Autodesk Inventor part; units mm, degrees
ref_plane "YZ Plane" through (0, 0, 0) normal (1, 0, 0) x (0, 1, 0)
ref_plane "XZ Plane" through (0, 0, 0) normal (0, 1, 0) x (-1, 0, 0)
ref_plane "XY Plane" through (0, 0, 0) normal (0, 0, 1) x (1, 0, 0)
ref_plane "Work Plane1" through (0, 0, 0) normal (0, 0, 1) x (1, 0, 0)
ref_plane "Work Plane2" through (0, 0, 0) normal (0, 0, 1) x (1, 0, 0)
sketch "Sketch3" plane through (0, 0, 0) normal (0, 0, 1) x (1, 0, 0)
  circle A0 centre (-75, -25) radius 100
  circle A1 centre (-75, -25) radius 95
  point P0 (-75, -25)
  point P1 (-75, -25)
  point P2 (-75, -25)
  point P3 (-75, -25)
extrude "Extrusion3" add sketch "Sketch3" along normal blind 3 contours A0 | A1
sketch "Sketch9" plane through (0, 0, 0) normal (0, 0, -1) x (-1, 0, 0)
  line L0 (115, -125) -> (35, -125)
  line L1 (35, -105) -> (95, -105)
  line L2 (95, -105) -> (95, -85)
  line L3 (95, -85) -> (35, -85)
  line L4 (35, -85) -> (35, -105)
  line L5 (35, -105) -> (95, -85) construction
  line L6 (95, -105) -> (35, -85) construction
  arc A0 (120.4545, -114.0724) -> (120.4545, 64.0724) centre (75, -25) ccw
  line L7 (85, -85) -> (85, -105)
  line L8 (45, -85) -> (45, -105)
  point P0 (0, 0)
  point P1 (105.3097, -125)
  point P2 (44.6903, -125)
  point P3 (65, -95)
  point P4 (111.3636, 68.1541)
  point P5 (111.3636, -118.1541)
  point P6 (95, -95)
  point P7 (85, -95)
  point P8 (35, -95)
  point P9 (45, -95)
  dimension "d48" = 60
  dimension "d49" = 20
  dimension "d53" = 10
  dimension "d54" = 10
  dimension "d56" = 20
  dimension "d57" = 20
extrude "Extrusion10" add sketch "Sketch9" along normal blind 20 contours L4 L3 L8 L1 | L7 L3 L2 L1
sketch "Sketch11" plane through (-45, -85, 0) normal (0, 1, 0) x (1, 0, 0)
  circle A0 centre (3.6, 4.915) radius 1.5
  line L0 (0, 20) -> (10, 20)
  line L1 (0, 0) -> (0, 20)
  circle A1 centre (-43.6, 4.915) radius 1.5
  line L2 (-50, 20) -> (-40, 20)
  line L3 (-40, 0) -> (-40, 20)
  line L4 (10, 0) -> (-70, 0)
  circle A2 centre (3.6, 15.085) radius 1.4068
  circle A3 centre (-43.6, 15.085) radius 1.5
  point P0 (45, 0)
  point P1 (5, 20)
  point P2 (0.3097, 0)
  point P3 (-60.3097, 0)
  dimension "d58" = 3
  dimension "d60" = 3.6
  dimension "d61" = 3
  dimension "d63" = 3.6
  dimension "d66" = 4.915
  dimension "d67" = 4.915
  dimension "d91" = 10.17
  dimension "d92" = 3
  dimension "d94" = 10.17
extrude "Extrusion12" cut sketch "Sketch11" against normal blind 20
sketch "Sketch12" plane through (0, 0, 0) normal (0, 0, -1) x (-1, 0, 0)
  line L0 (35, -105) -> (35, -85)
  line L1 (35, -85) -> (45, -85)
  line L2 (45, -85) -> (45, -105)
  line L3 (45, -105) -> (35, -105)
  line L4 (95, -85) -> (95, -105)
  line L5 (95, -105) -> (85, -105)
  line L6 (85, -105) -> (85, -85)
  line L7 (85, -85) -> (95, -85)
  circle A0 centre (75, -25) radius 11
  circle A1 centre (75, -25) radius 22
  circle A2 centre (75, -25) radius 100
  line L8 (75, -25) -> (92.5, -25)
  circle A3 centre (92.5, -25) radius 2.75
  line L9 (75, -25) -> (66.25, -9.8446)
  circle A4 centre (66.25, -9.8446) radius 2.75
  line L10 (75, -25) -> (66.25, -40.1554)
  circle A5 centre (66.25, -40.1554) radius 2.75
  point P0 (0, 0)
  point P1 (38.6364, 68.1541)
  point P2 (38.6364, -118.1541)
  dimension "d70" = 22
  dimension "d71" = 44
  dimension "d76" = 17.5
  dimension "d77" = 5.5
extrude "Extrusion13" cut sketch "Sketch12" against normal blind 35 contours L8 L9 A0 | A0 L10 L8 | L9 L10 A0
extrude "Extrusion14" cut sketch "Sketch12" against normal blind 2 contours A5 | A4 | A3 | A1
extrude "Extrusion15" cut sketch "Sketch12" against normal blind 3 contours A5 | A4 | A3
sketch "Sketch13" plane through (0, 0, 0) normal (0, 0, -1) x (-1, 0, 0)
  point P0 (0, 0)
sketch "Sketch14" plane through (0, 0, 0) normal (0, 0, -1) x (-1, 0, 0)
  line L0 (47, -80) -> (103, -80)
  line L1 (105, -78) -> (105, -57)
  line L2 (103, -55) -> (47, -55)
  line L3 (45, -57) -> (45, -78)
  line L4 (115, -125) -> (35, -125)
  circle A0 centre (75, -25) radius 11
  arc A1 (47, -55) -> (45, -57) centre (47, -57) ccw
  arc A2 (103, -80) -> (105, -78) centre (103, -78) ccw
  arc A3 (47, -55) -> (45, -57) centre (47, -57) ccw
  arc A4 (45, -78) -> (47, -80) centre (47, -78) ccw
  arc A5 (105, -57) -> (103, -55) centre (103, -57) ccw
  point P0 (0, 0)
  point P1 (105, -55)
  point P2 (105, -80)
  point P3 (45, -55)
  point P4 (105.3097, -125)
  point P5 (44.6903, -125)
  dimension "d84" = 60
  dimension "d85" = 25
  dimension "d86" = 45
  dimension "d87" = 30
  dimension "d88" = 2
extrude "Extrusion16" cut sketch "Sketch14" against normal blind 20 contours A4 L3 A1 L2 A5 L1 A2 L0
fillet "Fillet1" radius 5 4 edges at (-35, -95, -20) (-35, -95, 0) (-95, -95, 0) (-95, -95, -20)
properties part number "Pokrywa_góra"
Could you check a few things on this model? Use its own coordinates, in mm. A direction names the side the tool comes from. Coordinates: 2 decimals unless noted, no trailing zeros. Write each loop counter-clockwise with the first axis right and the second up, starting at its lowest first coordinate (ties: lowest second). Pieces come first, ordered by that corner, then holes. Notation, with made-up numbers: (12.25, 86.5) - (57.25, 86.5) arc R30 ccw to (57.25, 124.5) - close; hole circle Ø8 at (13, 27). An arc over 180 degrees is marked (long way). Put each result on its own line as item: value. Start each with the question number.
Q1. Please list where these lines run through material, in increasing order: L1, parallel to Z at x = -41.4, y = -94.5 (3 decimals); L2, parallel to Y at x = -66.25, z = 2.65; L3, parallel to Y at x = -64.5, z = 0.5.
Q2. I want a section at B-B on x = -60. Write out the boundary of the cut face in (y, z).
Q3. I want a section at D-D on y = 16.5. Write out the boundary of the cut face in (x, z).
Q4. I want a section at A-A on z = -11.25. Write out the boundary of the cut face in (x, y).
Q5. I'm going to push flat-ended pins straight in: P1, Ø5, axis at x = -88.6, z = -15.085, coming from the +Y side; P2, Ø5, axis at y = -102, z = -5, coming from the +X side; P3, Ø4.5, axis at x = -66.25, y = -40.16, coming from the -Z side; P4, Ø5, axis at y = -98, z = -9.5, coming from the -X side. Where does each tip first touch, or does it pass through?
Q6. Thinking about a two-plate mould opening in X: for faces 1 (the cylindrical face through (-33, -95, -1)), 2 (the flat face through (-87, -95, -20)), 3 (the cylindrical face through (-89.753, -24.879, 2.493)), which applies, pulls with the +X half, pulls with the -X half, needs draft (parallel to the pull), parting line crosses it, or undercut?
Q7. I want a section at C-C on y = -96.5. Write out the boundary of the cut face in (x, z) (3 decimals).
Q8. Which directions (+Z, -Z, +X, -X, +Y, -Y) give clear straight access to the entire face, cutting with the end or side of a thin tool? Please do faces 4 (the flat face through (-45, -95, -10)), 5 (the flat face through (-35, -95, -10)), 6 (the flat face through (-91, -85, -10)), 7 (the flat face through (-91, -105, -10)).
Checks:
1. L1: -20 to -16.492, -13.678 to -6.415, -3.415 to 3
1. L2: -124.62 to -80, -55 to -42.91, -37.41 to -31.67, -18.33 to -12.59, -7.09 to 74.62
1. L3: -124.45 to -80, -55 to -44.33, -5.67 to 74.45
2. outline: (-123.87, 0) - (-80, 0) - (-80, 3) - (-123.87, 3) - close; (-55, 0) - (-41.09, 0) - (-41.09, 2) - (-8.91, 2) - (-8.91, 0) - (73.87, 0) - (73.87, 3) - (-55, 3) - close
3. outline: (-165.98, 0) - (15.98, 0) - (15.98, 3) - (-165.98, 3) - close
4. outline: (-95, -105) - (-85, -105) - (-85, -85) - (-95, -85) - close; (-45, -105) - (-35, -105) - (-35, -85) - (-45, -85) - close
5. P1: y = -85
5. P2: x = -34.33
5. P3: through
5. P4: x = -95
6. face 1: pulls with the +X half
6. face 2: needs draft
6. face 3: undercut
7. outline: (-144.912, 0) - (-100, 0) arc R5 cw to (-95, -5) - (-95, -15) arc R5 ccw to (-90, -20) - (-85, -20) - (-85, 0) - (-45, 0) - (-45, -20) - (-40, -20) arc R5 ccw to (-35, -15) - (-35, -5) arc R5 cw to (-30, 0) - (-5.088, 0) - (-5.088, 3) - (-144.912, 3) - close; hole circle Ø3 at (-88.6, -15.085); hole circle Ø3 at (-88.6, -4.915); hole circle Ø3 at (-41.4, -4.915); hole circle Ø2.814 at (-41.4, -15.085)
8. face 4: -Z, +Y, -Y
8. face 5: -Z, +X, +Y, -Y
8. face 6: -Z, +X, -X, +Y
8. face 7: -Z, +X, -X, -Y
